from build123d import *

# Parameters (mm, degrees)
F1_DEPTH = 78.232


with BuildPart() as f1:
    # F0 (on Front) → F1 (new body)
    with BuildSketch(Plane.XZ):
        with BuildLine():
            ThreePointArc((-26.824391, 50.863773), (-30.883831, 53.534434), (-35.642884, 52.553162))
            ThreePointArc((-35.642884, 52.553162), (-27.260069, -57.351012), (63.257536, 5.543838))
            ThreePointArc((63.257536, 5.543838), (61.221431, 9.671485), (56.931782, 11.339454))
            Line((56.931782, 11.339454), (0, 11.339454))
            Line((0, 11.339454), (-26.824391, 50.863773))
        make_face()
    extrude(amount=F1_DEPTH)


solid = f1.part
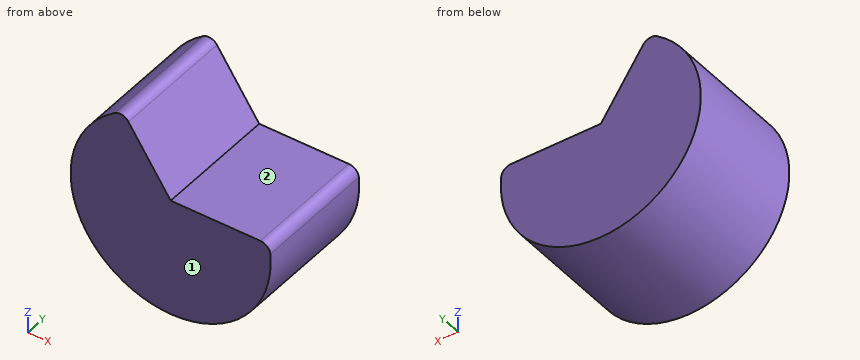
The model under review builds one solid part; all positions refer to its coordinate system, in mm. Face numbers are marked on the shaded views. A direction names the side the tool comes from. Give positions to 0.01 mm unless a question says otherwise; leave off trailing zeros. Order: outer loops, then holes, each group sorted by start corner. A loop starts at its lowest first (then second) coordinate and runs counter-clockwise, first axis right, second up. Notation, with made-up numbers: M 46,68.5 L 65,68.5 A14 ccw 65,86.5 Z; hole C 3,50 d2. An arc over 180 degrees is marked long. Use one line per item in the form item = value. Start each with the question number.
Item 1: For the marked faces 1 and 2, list the 3-axis set-ups (+Z, -Z, +X, -X, +Y, -Y) from which the entire face can be reached by the end or side of a thin tool; tool diameter is ignored.
Item 2: To check wall thickness, follow line 1 along Z through (x, y) = (-5, -71.5); line 2 along Z through (x, y) = (12.5, -35.5); line 3 along X through (y, z) = (-67.5, 2). State the ranges of each line that lie inside material, in increasing order. Write a range as from..to.
Item 3: We need section A-A on y = -6. Give the boundary of the cut face in (x, z), plus the area to 3 significant figures.
Item 4: Insertion check: pin 1 Ø1.5 at (x, y) = (-32, -67.5) entering from -Z; pin 2 Ø5 at (x, y) = (29, -10) entering from +Z; pin 3 Ø8 at (x, y) = (-13.5, -51.5) entering from +Z. Each pin has a flat end and moves straight along its axis. Give the tip position at first contact, or say it passes through.
Item 5: We need section B-B on x = 52. Give the boundary of the cut face in (y, z).
Item 6: We need section C-C on z = -51. Give the boundary of the cut face in (x, y).
Completed:
q1.face_1 = +Z, -Z, +X, -X, -Y
q1.face_2 = +Z, +X, +Y, -Y
q2.line_1 = -63.3..18.71
q2.line_2 = -62.26..11.34
q2.line_3 = -63.47..63.47
q3.outline = M -35.64,52.55 A63.5 ccw long 63.26,5.54 A6.35 ccw 56.93,11.34 L 0,11.34 L -26.82,50.86 A6.35 ccw Z
q3.area = 9,370 mm²
q4.pin_1 = -55.28
q4.pin_2 = 11.34
q4.pin_3 = 37.12
q5.outline = M -78.23,-36.45 L 0,-36.45 L 0,11.34 L -78.23,11.34 Z
q6.outline = M -37.83,-78.23 L 37.83,-78.23 L 37.83,0 L -37.83,0 Z
